The model under review builds one solid part; all positions refer to its coordinate system, in mm. Face numbers are marked on the shaded views. Round coordinates to 2 decimals unless told otherwise and drop trailing zeros. Write each loop counter-clockwise with the first axis right and the second up, starting at its lowest first coordinate (ties: lowest second). Pieces come first, ordered by that corner, then holes. Notation, with made-up numbers: (-29.75, 61) - (-14.75, 61) arc R31 cw to (-14.75, 98) - close; hole circle Ø10 at (26, 62.5). An arc over 180 degrees is marked (long way). Return JSON: item names as keys, results as strings.
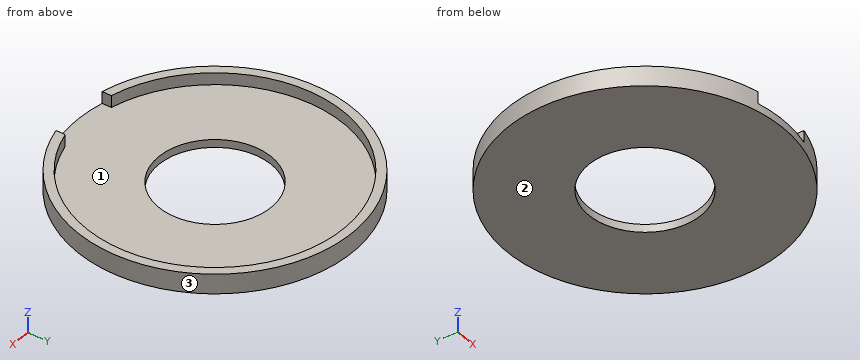
Autodesk Inventor part; units mm, degrees
ref_plane "YZ Plane" through (0, 0, 0) normal (1, 0, 0) x (0, 1, 0)
ref_plane "XZ Plane" through (0, 0, 0) normal (0, 1, 0) x (-1, 0, 0)
ref_plane "XY Plane" through (0, 0, 0) normal (0, 0, 1) x (1, 0, 0)
sketch "Skizze1" plane through (0, 0, 0) normal (0, 0, 1) x (1, 0, 0)
  circle A0 centre (0, 0) radius 34.775
  dimension "d0" = 69.55
extrude "Extrusion1" add sketch "Skizze1" along normal blind 5
sketch "Skizze2" plane through (0, 0, 5) normal (0, 0, 1) x (1, 0, 0)
  circle A0 centre (0, 0) radius 32.54
  dimension "d3" = 65.08
extrude "Extrusion2" cut sketch "Skizze2" against normal blind 3
sketch "Skizze3" plane through (0, 0, 0) normal (0, 0, -1) x (-1, 0, 0)
  circle A0 centre (0, 0) radius 14.195
  dimension "d6" = 28.39
extrude "Extrusion3" cut sketch "Skizze3" against normal through all
sketch "Skizze4" plane through (0, 0, 5) normal (0, 0, 1) x (1, 0, 0)
  line L0 (-8, -42.775) -> (8, -42.775)
  line L1 (8, -42.775) -> (8, -26.775)
  line L2 (8, -26.775) -> (-8, -26.775)
  line L3 (-8, -26.775) -> (-8, -42.775)
  circle A0 centre (0, 0) radius 34.775
  line L4 (-8, -42.775) -> (8, -26.775) construction
  line L5 (8, -42.775) -> (-8, -26.775) construction
  point P0 (0, -34.775)
  dimension "d9" = 16
  dimension "d10" = 16
extrude "Extrusion4" cut sketch "Skizze4" against normal up to surface (3 mm away) contours L3 A0 L1 L0 | L3 L2 L1 A0 picked at (0.896, -29.407)
properties part number "2024_08_28_Holder_disk_GL25"
(1) Add section D-D (y = 24.5). Write out the cut boundary in (x, z), plus the area to 3 significant figures.
Filled in:
{"outline": "(-24.68, 0) - (24.68, 0) - (24.68, 5) - (21.41, 5) - (21.41, 2) - (-21.41, 2) - (-21.41, 5) - (-24.68, 5) - close", "area": "118 mm2"}
(2) Wall thickness on line 1 (Y direction, x = 0, z = 1.65) (3 decimals); line 2 (X direction, y = 0, z = 3.25) (3 decimals); line 3 (Z direction, x = -6.5, y = 23): over which ranges is each line inside the solid? List them lowest first.
Filled in:
{"line 1": "y = -34.775 to -14.195, 14.195 to 34.775", "line 2": "x = -34.775 to -32.54, 32.54 to 34.775", "line 3": "z = 0 to 2"}
(3) Add section B-B (x = 0). Write out the cut boundary in (y, z) (3 decimals), plus the area to 3 significant figures.
Filled in:
{"outline": "(-34.775, 0) - (-14.195, 0) - (-14.195, 2) - (-34.775, 2) - close; (14.195, 0) - (34.775, 0) - (34.775, 5) - (32.54, 5) - (32.54, 2) - (14.195, 2) - close", "area": "89.0 mm2"}
(4) Add section C-C (x = -22). Write out the cut boundary in (y, z).
Filled in:
{"outline": "(-26.93, 0) - (26.93, 0) - (26.93, 5) - (23.98, 5) - (23.98, 2) - (-23.98, 2) - (-23.98, 5) - (-26.93, 5) - close"}
(5) Add section A-A (y = 0). Write out the cut boundary in (x, z) (3 decimals).
Filled in:
{"outline": "(-34.775, 0) - (-14.195, 0) - (-14.195, 2) - (-32.54, 2) - (-32.54, 5) - (-34.775, 5) - close; (14.195, 0) - (34.775, 0) - (34.775, 5) - (32.54, 5) - (32.54, 2) - (14.195, 2) - close"}
(6) Clearance check with flat-ended pins moving along their axes: pin 1 Ø1 at (x, y) = (24, 0.5) entering from +Z; pin 2 Ø1.2 at (y, z) = (-32.5, 4) entering from -X; pin 3 Ø3 at (y, z) = (-6, 4) entering from -X. State where each tip first meets the part, or that it passes through.
Filled in:
{"pin 1": "stops at z = 2", "pin 2": "stops at x = -13.85", "pin 3": "stops at x = -34.48"}
(7) Mouldability with a two-part tool opening along Y and no side actions: class the marked faces 1, 2 and 3 as released by +Y, released by -Y, zero draft, split by the parting line, or undercut.
Filled in:
{"face 1": "undercut", "face 2": "zero draft", "face 3": "split by the parting line"}
